Can you work these out from the model? Positions are in its coordinate system, mm. A direction names the side the tool comes from. Coordinates: 2 decimals unless noted, no trailing zeros. Order: outer loops, then holes, each group sorted by start corner. A loop starts at its lowest first (then second) coordinate and runs counter-clockwise, first axis right, second up. Notation, with made-up numbers: M 86,-10.5 L 106,-10.5 A17 ccw 106,21.5 Z; hole C 27.5,60.25 d6. An arc over 180 degrees is marked long. Answer as a JSON object with one key per item and string values.
Autodesk Inventor part; units mm, degrees
ref_plane "YZ Plane" through (0, 0, 0) normal (1, 0, 0) x (0, 1, 0)
ref_plane "XZ Plane" through (0, 0, 0) normal (0, 1, 0) x (-1, 0, 0)
ref_plane "XY Plane" through (0, 0, 0) normal (0, 0, 1) x (1, 0, 0)
sketch "Sketch1" plane through (0, 0, 0) normal (0, 0, 1) x (1, 0, 0)
  point P0 (0, 0)
sketch "Sketch2" plane through (0, 0, 0) normal (0, 0, 1) x (1, 0, 0)
  line L0 (0, 0) -> (20.4, 0)
  line L1 (20.4, 0) -> (20.4, 21.7)
  line L2 (20.4, 21.7) -> (0, 21.7)
  line L3 (0, 21.7) -> (0, 0)
  line L4 (40, 0) -> (60.4, 0)
  line L5 (60.4, 0) -> (60.4, 21.7)
  line L6 (60.4, 21.7) -> (40, 21.7)
  line L7 (40, 21.7) -> (40, 0)
  line L8 (80, 0) -> (100.4, 0)
  line L9 (100.4, 0) -> (100.4, 21.7)
  line L10 (100.4, 21.7) -> (80, 21.7)
  line L11 (80, 21.7) -> (80, 0)
  line L12 (0, -40) -> (20.4, -40)
  line L13 (20.4, -40) -> (20.4, -18.3)
  line L14 (20.4, -18.3) -> (0, -18.3)
  line L15 (0, -18.3) -> (0, -40)
  line L16 (40, -40) -> (60.4, -40)
  line L17 (60.4, -40) -> (60.4, -18.3)
  line L18 (60.4, -18.3) -> (40, -18.3)
  line L19 (40, -18.3) -> (40, -40)
  line L20 (80, -40) -> (100.4, -40)
  line L21 (100.4, -40) -> (100.4, -18.3)
  line L22 (100.4, -18.3) -> (80, -18.3)
  line L23 (80, -18.3) -> (80, -40)
  line L24 (100.4, 21.7) -> (175.4, 21.7) construction
  line L25 (175.4, 21.7) -> (175.4, -53.3) construction
  line L26 (175.4, -53.3) -> (100.4, -53.3) construction
  line L27 (100.4, -53.3) -> (100.4, 21.7) construction
  circle A0 centre (115.4, 15.1) radius 6.6 construction
  line L28 (115.4, 15.1) -> (115.4, -53.3) construction
  circle A1 centre (115.4, -8.9) radius 6.6 construction
  circle A2 centre (115.4, -32.9) radius 6.6 construction
  line L29 (100.4, 15.1) -> (200.3961, 15.1) construction
  circle A3 centre (139.4, 15.1) radius 6.6 construction
  circle A4 centre (139.4, -8.9) radius 6.6 construction
  circle A5 centre (139.4, -32.9) radius 6.6 construction
  circle A6 centre (115.4, 15.1) radius 6.6
  circle A7 centre (139.4, 15.1) radius 6.6 construction
  circle A8 centre (139.4, 15.1) radius 6.6
  circle A9 centre (115.4, -8.9) radius 6.6 construction
  circle A10 centre (115.4, -8.9) radius 6.6
  circle A11 centre (139.4, -8.9) radius 6.6 construction
  circle A12 centre (139.4, -8.9) radius 6.6
  circle A13 centre (115.4, -32.9) radius 6.6 construction
  circle A14 centre (115.4, -32.9) radius 6.6
  circle A15 centre (139.4, -32.9) radius 6.6 construction
  circle A16 centre (139.4, -32.9) radius 6.6
  line L30 (0, 21.7) -> (-12, 21.7) construction
  line L31 (-12, 21.7) -> (-12, 33.7) construction
  line L32 (-12, 33.7) -> (0, 33.7) construction
  line L33 (0, 33.7) -> (0, 21.7) construction
  line L34 (146, -40) -> (158, -40) construction
  line L35 (158, -40) -> (158, -52) construction
  line L36 (158, -52) -> (146, -52) construction
  line L37 (146, -52) -> (146, -40) construction
  line L38 (139.4, -32.9) -> (139.4, -74.4589) construction
  line L39 (-12, 33.7) -> (158, 33.7)
  line L40 (158, 33.7) -> (158, -52)
  line L41 (158, -52) -> (-12, -52)
  line L42 (-12, -52) -> (-12, 33.7)
  point P0 (146, -46)
  dimension "d0" = 20.4
  dimension "d1" = 21.7
  dimension "d5" = 40
  dimension "d8" = 40
  dimension "d11" = 75
  dimension "d12" = 75
  dimension "d13" = 13.2
  dimension "d14" = 15
  dimension "d15" = 13.2
  dimension "d16" = 24
  dimension "d17" = 13.2
  dimension "d18" = 24
  dimension "d19" = 61.7
  dimension "d20" = 13.2
  dimension "d21" = 24
  dimension "d22" = 13.2
  dimension "d23" = 13.2
  dimension "d26" = 24
  dimension "d29" = 24
  dimension "d32" = 12
  dimension "d33" = 12
  dimension "d34" = 12
  dimension "d35" = 12
  dimension "d36" = 6.6
extrude "Extrusion1" add sketch "Sketch2" along normal blind 2.5
sketch "Sketch3" plane through (0, 0, 2.5) normal (0, 0, 1) x (1, 0, 0)
  line L0 (-12, -52) -> (158, -52) construction
  line L1 (158, -52) -> (158, 33.7) construction
  line L2 (158, 33.7) -> (-12, 33.7) construction
  line L3 (-12, 33.7) -> (-12, -52) construction
  circle A0 centre (115.4, 15.1) radius 6.6 construction
  circle A1 centre (139.4, 15.1) radius 6.6 construction
  circle A2 centre (115.4, -8.9) radius 6.6 construction
  circle A3 centre (139.4, -8.9) radius 6.6 construction
  circle A4 centre (115.4, -32.9) radius 6.6 construction
  circle A5 centre (139.4, -32.9) radius 6.6 construction
  line L4 (80, -40) -> (80, -18.3) construction
  line L5 (80, -18.3) -> (100.4, -18.3) construction
  line L6 (100.4, -18.3) -> (100.4, -40) construction
  line L7 (100.4, -40) -> (80, -40) construction
  line L8 (40, -40) -> (40, -18.3) construction
  line L9 (40, -18.3) -> (60.4, -18.3) construction
  line L10 (60.4, -18.3) -> (60.4, -40) construction
  line L11 (60.4, -40) -> (40, -40) construction
  line L12 (0, -40) -> (0, -18.3) construction
  line L13 (0, -18.3) -> (20.4, -18.3) construction
  line L14 (20.4, -18.3) -> (20.4, -40) construction
  line L15 (20.4, -40) -> (0, -40) construction
  line L16 (80, 0) -> (80, 21.7) construction
  line L17 (80, 21.7) -> (100.4, 21.7) construction
  line L18 (100.4, 21.7) -> (100.4, 0) construction
  line L19 (100.4, 0) -> (80, 0) construction
  line L20 (40, 0) -> (40, 21.7) construction
  line L21 (40, 21.7) -> (60.4, 21.7) construction
  line L22 (60.4, 21.7) -> (60.4, 0) construction
  line L23 (60.4, 0) -> (40, 0) construction
  line L24 (0, 0) -> (0, 21.7) construction
  line L25 (0, 21.7) -> (20.4, 21.7) construction
  line L26 (20.4, 21.7) -> (20.4, 0) construction
  line L27 (20.4, 0) -> (0, 0) construction
  line L28 (-7, 28.7) -> (153, 28.7) construction
  line L29 (153, 28.7) -> (153, -47) construction
  line L30 (153, -47) -> (-7, -47) construction
  line L31 (-7, -47) -> (-7, 28.7) construction
  line L32 (-7, -9.15) -> (-7, -6.65) construction
  line L33 (-7, -6.65) -> (-7, -11.65) construction
  line L34 (20.4, 21.7) -> (40, 21.7) construction
  line L35 (30.2, 21.7) -> (30.2, 28.7) construction
  line L36 (60.4, 21.7) -> (80, 21.7) construction
  line L37 (70.2, 21.7) -> (70.2, 28.7) construction
  line L38 (30.2, 28.7) -> (32.7, 28.7) construction
  line L39 (70.2, 28.7) -> (72.7, 28.7) construction
  line L40 (32.7, 28.7) -> (27.7, 28.7) construction
  line L41 (27.7, 28.7) -> (27.7, -47) construction
  line L42 (27.7, -47) -> (32.7, -47) construction
  line L43 (32.7, -47) -> (32.7, 28.7) construction
  line L44 (72.7, 28.7) -> (67.7, 28.7) construction
  line L45 (67.7, 28.7) -> (67.7, -47) construction
  line L46 (67.7, -47) -> (72.7, -47) construction
  line L47 (72.7, -47) -> (72.7, 28.7) construction
  circle A6 centre (115.4, 15.1) radius 6.6 construction
  line L48 (108.8, 15.1) -> (100.4, 15.1) construction
  line L49 (104.6, 15.1) -> (104.6, 28.7) construction
  line L50 (104.6, 28.7) -> (106.6, 28.7) construction
  line L51 (106.6, 28.7) -> (102.6, 28.7) construction
  line L52 (102.6, 28.7) -> (102.6, -47) construction
  line L53 (102.6, -47) -> (106.6, -47) construction
  line L54 (106.6, -47) -> (106.6, 28.7) construction
  line L55 (-7, -6.65) -> (-7, -11.65) construction
  line L56 (-7, -11.65) -> (106.6, -11.65) construction
  line L57 (106.6, -11.65) -> (106.6, -6.65) construction
  line L58 (106.6, -6.65) -> (-7, -6.65) construction
  line L59 (115.4, -2.3) -> (115.4, 8.5) construction
  line L60 (122, 15.1) -> (132.8, 15.1) construction
  line L61 (115.4, -26.3) -> (115.4, -15.5) construction
  line L62 (106.6, 3.1) -> (106.6, 1.1) construction
  line L63 (106.6, 1.1) -> (106.6, 5.1) construction
  line L64 (106.6, 5.1) -> (153, 5.1) construction
  line L65 (153, 5.1) -> (153, 1.1) construction
  line L66 (153, 1.1) -> (106.6, 1.1) construction
  line L67 (106.6, -20.9) -> (106.6, -22.9) construction
  line L68 (106.6, -22.9) -> (106.6, -18.9) construction
  line L69 (106.6, -18.9) -> (153, -18.9) construction
  line L70 (153, -18.9) -> (153, -22.9) construction
  line L71 (153, -22.9) -> (106.6, -22.9) construction
  line L72 (127.4, 28.7) -> (129.4, 28.7) construction
  line L73 (129.4, 28.7) -> (125.4, 28.7) construction
  line L74 (125.4, 28.7) -> (125.4, -47) construction
  line L75 (125.4, -47) -> (129.4, -47) construction
  line L76 (129.4, -47) -> (129.4, 28.7) construction
  line L77 (-7, -11.65) -> (106.6, -11.65)
  line L78 (106.6, -11.65) -> (106.6, -6.65)
  line L79 (106.6, -6.65) -> (-7, -6.65)
  line L80 (-7, -6.65) -> (-7, -11.65)
  line L81 (102.6, 28.7) -> (106.6, 28.7)
  line L82 (106.6, 28.7) -> (106.6, -47)
  line L83 (106.6, -47) -> (102.6, -47)
  line L84 (102.6, -47) -> (102.6, 28.7)
  line L85 (125.4, -47) -> (129.4, -47)
  line L86 (129.4, -47) -> (129.4, 28.7)
  line L87 (129.4, 28.7) -> (125.4, 28.7)
  line L88 (125.4, 28.7) -> (125.4, -47)
  line L89 (102.6, 5.1) -> (153, 5.1)
  line L90 (153, 5.1) -> (153, 1.1)
  line L91 (153, 1.1) -> (102.6, 1.1)
  line L92 (102.6, 1.1) -> (102.6, 5.1)
  line L93 (153, -18.9) -> (102.6, -18.9)
  line L94 (102.6, -18.9) -> (102.6, -22.9)
  line L95 (102.6, -22.9) -> (153, -22.9)
  line L96 (153, -22.9) -> (153, -18.9)
  line L97 (67.7, 28.7) -> (72.7, 28.7)
  line L98 (72.7, 28.7) -> (72.7, -47)
  line L99 (72.7, -47) -> (67.7, -47)
  line L100 (67.7, -47) -> (67.7, 28.7)
  line L101 (32.7, 28.7) -> (27.7, 28.7)
  line L102 (27.7, 28.7) -> (27.7, -47)
  line L103 (27.7, -47) -> (32.7, -47)
  line L104 (32.7, -47) -> (32.7, 28.7)
  line L105 (27.7, 28.7) -> (32.7, 28.7)
  line L106 (32.7, 28.7) -> (32.7, 33.7)
  line L107 (32.7, 33.7) -> (27.7, 33.7)
  line L108 (27.7, 33.7) -> (27.7, 28.7)
  line L109 (158, 33.7) -> (-12, 33.7)
  line L110 (67.7, 28.7) -> (72.7, 28.7)
  line L111 (72.7, 28.7) -> (72.7, 33.7)
  line L112 (72.7, 33.7) -> (67.7, 33.7)
  line L113 (67.7, 33.7) -> (67.7, 28.7)
  line L114 (102.6, 28.7) -> (106.6, 28.7)
  line L115 (106.6, 28.7) -> (106.6, 33.7)
  line L116 (106.6, 33.7) -> (102.6, 33.7)
  line L117 (102.6, 33.7) -> (102.6, 28.7)
  line L118 (125.4, 28.7) -> (129.4, 28.7)
  line L119 (129.4, 28.7) -> (129.4, 33.7)
  line L120 (129.4, 33.7) -> (125.4, 33.7)
  line L121 (125.4, 33.7) -> (125.4, 28.7)
  point P0 (102.6, -6.65)
  point P1 (72.7, -6.65)
  point P2 (67.7, -6.65)
  point P3 (32.7, -6.65)
  point P4 (27.7, -6.65)
  point P5 (27.7, -11.65)
  point P6 (32.7, -11.65)
  point P7 (67.7, -11.65)
  point P8 (72.7, -11.65)
  point P9 (102.6, -11.65)
  point P10 (125.4, -22.9)
  point P11 (129.4, -22.9)
  point P12 (129.4, -18.9)
  point P13 (129.4, 1.1)
  point P14 (129.4, 5.1)
  point P15 (125.4, 5.1)
  point P16 (106.6, 5.1)
  point P17 (125.4, 1.1)
  point P18 (125.4, -18.9)
  dimension "d39" = 5
  dimension "d40" = 2.5
  dimension "d42" = 2.5
  dimension "d43" = 2.5
  dimension "d44" = 5
  dimension "d45" = 5
  dimension "d46" = 2
  dimension "d47" = 4
  dimension "d48" = 5
  dimension "d49" = 2
  dimension "d50" = 4
  dimension "d51" = 2
  dimension "d52" = 4
  dimension "d53" = 2
  dimension "d54" = 4
extrude "Extrusion2" add sketch "Sketch3" along normal blind 4 contours L80 L79 L102 L77 | L102 L79 L104 L77 | L77 L104 L103 L102 | L104 L79 L100 L77 | L102 L101 L104 L79 | L100 L79 L98 L77 | L77 L98 L99 L100 | L108 L107 L106 L101 | L98 L79 L84 L77 | L100 L97 L98 L79 | L84 L79 L78 L77 | L77 L82 L93 L84 | L113 L109 L111 L97 | L93 L82 L95 L84 | L84 L91 L82 L79 | L93 L88 L95 L82 | L95 L82 L83 L84 | L84 L89 L82 L91 | L82 L89 L88 L91 | L93 L86 L95 L88 | L88 L91 L86 L93 | L84 L81 L82 L89 | L109 L115 L81 L117 | L88 L89 L86 L91 | L95 L86 L85 L88 | L93 L96 L95 L86 | L88 L87 L86 L89 | L86 L89 L90 L91 | L109 L119 L87 L121
properties part number "faceplate"
Item 1: I want a section at A-A, the plane y = -8.9. Write out the boundary of the cut face in (x, z).
Answers follow:
{"outline": "M -12,0 L 108.8,0 L 108.8,2.5 L 106.6,2.5 L 106.6,6.5 L -7,6.5 L -7,2.5 L -12,2.5 Z; M 122,0 L 132.8,0 L 132.8,2.5 L 129.4,2.5 L 129.4,6.5 L 125.4,6.5 L 125.4,2.5 L 122,2.5 Z; M 146,0 L 158,0 L 158,2.5 L 146,2.5 Z"}
Item 2: Please list where these lines run through material, in increasing order: line 1 (X direction, y = -28, z = 4.75); line 2 (Y direction, x = 139.4, z = 0.85); line 3 (Y direction, x = 18.5, z = 0.75).
Answers follow:
{"line 1": "x = 27.7 to 32.7, 67.7 to 72.7, 102.6 to 106.6, 125.4 to 129.4", "line 2": "y = -52 to -39.5, -26.3 to -15.5, -2.3 to 8.5, 21.7 to 33.7", "line 3": "y = -52 to -40, -18.3 to 0, 21.7 to 33.7"}
Item 3: Which directions (+Z, -Z, +X, -X, +Y, -Y) give clear straight access to the entire face, cutting with the end or side of a thin tool? Please do faces 1 (the flat face through (72.7, 14, 4)), 2 (the flat face through (32.7, -30, 4)), 3 (the flat face through (70, -47, 4)), 4 (the flat face through (141, -18.9, 4)).
Answers follow:
{"face 1": "+Z, +Y", "face 2": "+Z, -Y", "face 3": "+Z, +X, -X, -Y", "face 4": "+Z, +X"}
Item 4: I want a section at C-C, the plane x = 24.5. Write out the boundary of the cut face in (y, z), plus the area to 3 significant figures.
Answers follow:
{"outline": "M -52,0 L 33.7,0 L 33.7,2.5 L -6.65,2.5 L -6.65,6.5 L -11.65,6.5 L -11.65,2.5 L -52,2.5 Z", "area": "234 mm^2"}
Item 5: If we mould it in two halves opening along Y, with no side actions, what happens to faces 5 (the cylindrical face through (121.497, -30.372, 1.232)), 6 (the flat face through (116, 5.1, 4)), 7 (the flat face through (67.7, 13, 4)), 8 (the flat face through (105, -47, 4))? For each: pulls with the +Y half, pulls with the -Y half, needs draft (parallel to the pull), parting line crosses it, or undercut.
Answers follow:
{"face 5": "undercut", "face 6": "pulls with the +Y half", "face 7": "needs draft", "face 8": "pulls with the -Y half"}
Item 6: I want a section at D-D, the plane y = 15.1. Give the number of separate pieces and of enclosed holes in the cut face, plus the area to 3 significant figures.
Answers follow:
{"separate pieces": "6", "enclosed holes": "0", "area": "278 mm^2"}
Item 7: I'm going to push flat-ended pins straight in: pin 1 (1.5 mm diameter, centred on y = -15.5, z = 4.5, fed in from -X); pin 2 (1.2 mm diameter, centred on y = 6.5, z = 3.5, fed in from +X); pin 3 (3 mm diameter, centred on x = 38.5, z = 5, fed in from +Y); pin 4 (10 mm diameter, centred on x = 73.5, y = -21.5, fed in from -Z). Where does each tip first touch, or does it pass through?
Answers follow:
{"pin 1": "stops at x = 27.7", "pin 2": "stops at x = 129.4", "pin 3": "stops at y = -6.65", "pin 4": "stops at z = 0"}
Item 8: I want a section at B-B, the plane x = 139.4. Write out the boundary of the cut face in (y, z).
Answers follow:
{"outline": "M -52,0 L -39.5,0 L -39.5,2.5 L -52,2.5 Z; M -26.3,0 L -15.5,0 L -15.5,2.5 L -18.9,2.5 L -18.9,6.5 L -22.9,6.5 L -22.9,2.5 L -26.3,2.5 Z; M -2.3,0 L 8.5,0 L 8.5,2.5 L 5.1,2.5 L 5.1,6.5 L 1.1,6.5 L 1.1,2.5 L -2.3,2.5 Z; M 21.7,0 L 33.7,0 L 33.7,2.5 L 21.7,2.5 Z"}
